Input: part model. Units: mm. Frame: model coordinates. A direction names the side the tool comes from. Coordinates: 2 decimals unless noted, no trailing zeros. Write each loop counter-clockwise with the first axis right and the second up, starting at its lowest first coordinate (ties: lowest second). Pieces come first, ordered by that corner, then holes. Notation, with made-up numbers: (75.25, -18) - (85.25, -18) arc R20 cw to (85.25, 1) - close; hole circle Ø8 at (-32.75, -38). An arc over 180 degrees is marked (long way). Put each result on its own line as item: value. Start each with the question number.
1. Cut plane A-A, the plane x = -21.25. Return loops of the section in (y, z).
2. Access query for faces 5 (the flat face through (-45, 40.364, 1)), 6 (the flat face through (-26.813, 36.211, 0.986)), 7 (the flat face through (-30.617, 37.276, 0.986)). Directions: +Z, -Z, +X, -X, +Y, -Y. A direction counts if a zero-diameter tool reaches every point of the face in a straight line with its end or side. Return the directions, or none.
3. Cut plane B-B, the plane z = 0.7. Count the separate pieces of the cut face and the enclosed holes in it, and give its area (3 significant figures).
4. Pull-direction query (Y, two-part tool) for faces 1 (the flat face through (-30, 34, 0)), 2 (the flat face through (-31, 32.172, 1)), 3 (the flat face through (-23.75, 34.6, 0.99)), 4 (the flat face through (-37.9, 36.33, 0.99)); classes: released by +Y, released by -Y, zero draft, split by the parting line, or undercut.
5. Pin query (flat end, axial travel): pin 1 (1 mm diameter, centred on y = 36, z = 1.5, fed in from +X); pin 2 (1 mm diameter, centred on x = -42.5, y = 37.5, fed in from -Z). Return the tip coordinate at first contact, or that it passes through.
6. Cut plane D-D, the plane x = -30.5. Return loops of the section in (y, z).
7. Line query: line 1 (X direction, y = 39.25, z = 0.6); line 2 (Y direction, x = -43, z = 0.4); line 3 (X direction, y = 31.5, z = 0.9). Output: solid intervals per line, ascending.
from build123d import *

# Parameters (mm, degrees)
BOSS_EXTRUDE1_DEPTH = 2


with BuildPart() as part:
    # Sketch1 → Boss-Extrude1 (new body)
    with BuildSketch(Plane.XY):
        with BuildLine():
            Line((-18.745582546, 31.006914048), (-21.79105099, 40.364252392))
            Line((-21.79105099, 40.364252392), (-23.123022137, 40.364252392))
            Line((-23.123022137, 40.364252392), (-25.740106044, 32.171592169))
            Line((-25.740106044, 32.171592169), (-28.102880037, 32.171592169))
            Line((-28.102880037, 32.171592169), (-25.485755278, 40.364252392))
            Line((-25.485755278, 40.364252392), (-26.78426782, 40.364252392))
            Line((-26.78426782, 40.364252392), (-28.598181785, 34.273274652))
            add(Edge.make_bspline(
                [(-28.598181785, 34.273274652), (-28.792274379, 33.597239241), (-28.906090832, 33.19565427), (-29.126942139, 32.251909163)],
                knots=[6, 6, 6, 6, 7, 7, 7, 7], degree=3))
            add(Edge.make_bspline(
                [(-29.126942139, 32.251909163), (-29.414792363, 33.316129761), (-29.448250968, 33.490163533), (-29.695901842, 34.273274652)],
                knots=[7, 7, 7, 7, 8, 8, 8, 8], degree=3))
            Line((-29.695901842, 34.273274652), (-31.563333235, 40.364252392))
            Line((-31.563333235, 40.364252392), (-32.861845777, 40.364252392))
            Line((-32.861845777, 40.364252392), (-30.197903482, 32.171592169))
            Line((-30.197903482, 32.171592169), (-32.614194903, 32.171592169))
            Line((-32.614194903, 32.171592169), (-35.278137198, 40.364252392))
            Line((-35.278137198, 40.364252392), (-36.610149199, 40.364252392))
            Line((-36.610149199, 40.364252392), (-39.227233105, 32.171592169))
            Line((-39.227233105, 32.171592169), (-40.519045756, 32.171592169))
            add(Edge.make_bspline(
                [(-40.519045756, 32.171592169), (-40.257995098, 32.593235961), (-40.110760894, 33.122037168), (-40.110760894, 33.69765591)],
                knots=[16, 16, 16, 16, 17, 17, 17, 17], degree=3))
            add(Edge.make_bspline(
                [(-40.110760894, 33.69765591), (-40.110760894, 34.82213468), (-40.572604036, 35.511569875), (-41.583307207, 35.913154846)],
                knots=[17, 17, 17, 17, 18, 18, 18, 18], degree=3))
            add(Edge.make_bspline(
                [(-41.583307207, 35.913154846), (-40.739937916, 36.374997988), (-40.365111659, 37.010874903), (-40.365111659, 37.947920118)],
                knots=[18, 18, 18, 18, 19, 19, 19, 19], degree=3))
            add(Edge.make_bspline(
                [(-40.365111659, 37.947920118), (-40.365111659, 38.764530696), (-40.679679744, 39.433866215), (-41.261998378, 39.842151078)],
                knots=[19, 19, 19, 19, 20, 20, 20, 20], degree=3))
            add(Edge.make_bspline(
                [(-41.261998378, 39.842151078), (-41.790799584, 40.23707701), (-42.353018543, 40.364252392), (-43.477497314, 40.364252392)],
                knots=[20, 20, 20, 20, 21, 21, 21, 21], degree=3))
            Line((-43.477497314, 40.364252392), (-46.817515873, 40.364252392))
            Line((-46.817515873, 40.364252392), (-46.817515873, 31.006914048))
            Line((-46.817515873, 31.006914048), (-18.745582546, 31.006914048))
        make_face()
        with BuildLine():
            Line((-43.142829554, 32.171592169), (-45.652837753, 32.171592169))
            Line((-45.652837753, 32.171592169), (-45.652837753, 35.257219109))
            Line((-45.652837753, 35.257219109), (-43.008995132, 35.257219109))
            add(Edge.make_bspline(
                [(-43.008995132, 35.257219109), (-41.958133464, 35.257219109), (-41.362415047, 34.708359081), (-41.362415047, 34.051267898), (-41.362415047, 33.725531232), (-41.362415054, 33.724414624)],
                knots=[0, 0, 0, 0, 1, 2, 2.003439864, 2.003439864, 2.003439864, 2.003439864], degree=3))
            add(Edge.make_bspline(
                [(-41.362415054, 33.724414624), (-41.362417047, 33.400922858), (-41.363577782, 32.75955684), (-42.038450458, 32.171592169), (-43.142829554, 32.171592169)],
                knots=[2.003439864, 2.003439864, 2.003439864, 2.003439864, 3, 4, 4, 4, 4], degree=3))
        make_face(mode=Mode.SUBTRACT)
        with BuildLine():
            Line((-33.87924884, 32.171592169), (-37.955479277, 32.171592169))
            Line((-37.955479277, 32.171592169), (-36.489632855, 37.091191897))
            add(Edge.make_bspline(
                [(-36.489632855, 37.091191897), (-36.295540261, 37.767227308), (-36.181764662, 38.17551217), (-35.960872501, 39.112598239)],
                knots=[1, 1, 1, 1, 2, 2, 2, 2], degree=3))
            add(Edge.make_bspline(
                [(-35.960872501, 39.112598239), (-35.679763022, 38.048336787), (-35.639604525, 37.881002907), (-35.391953651, 37.091191897)],
                knots=[2, 2, 2, 2, 3, 3, 3, 3], degree=3))
            Line((-35.391953651, 37.091191897), (-33.87924884, 32.171592169))
        make_face(mode=Mode.SUBTRACT)
        with BuildLine():
            add(Edge.make_bspline(
                [(-22.47374544, 39.112598239), (-22.19263596, 38.048336787), (-22.152477463, 37.881002907), (-21.904826589, 37.091191897)],
                knots=[1, 1, 1, 1, 2, 2, 2, 2], degree=3))
            Line((-21.904826589, 37.091191897), (-20.392121778, 32.171592169))
            Line((-20.392121778, 32.171592169), (-24.47509296, 32.171592169))
            Line((-24.47509296, 32.171592169), (-23.009246538, 37.091191897))
            add(Edge.make_bspline(
                [(-23.009246538, 37.091191897), (-22.808413199, 37.767227308), (-22.6946376, 38.17551217), (-22.47374544, 39.112598239)],
                knots=[0, 0, 0, 0, 1, 1, 1, 1], degree=3))
        make_face(mode=Mode.SUBTRACT)
        with BuildLine():
            Line((-45.652837753, 36.348239275), (-45.652837753, 39.199615125))
            Line((-45.652837753, 39.199615125), (-43.336963001, 39.199615125))
            add(Edge.make_bspline(
                [(-43.336963001, 39.199615125), (-42.7278448, 39.199615125), (-42.37024646, 39.09102995), (-42.179170008, 38.931701151), (-42.093373815, 38.855654373)],
                knots=[0, 0, 0, 0, 1, 1.908075185, 1.908075185, 1.908075185, 1.908075185], degree=3))
            add(Edge.make_bspline(
                [(-42.093373815, 38.855654373), (-42.083891518, 38.847731554), (-42.074504957, 38.839663032), (-42.065209172, 38.831447907)],
                knots=[1.967701589, 1.967701589, 1.967701589, 1.967701589, 2, 2, 2, 2], degree=3))
            add(Edge.make_bspline(
                [(-42.065209172, 38.831447907), (-42.05671789, 38.823784642), (-42.048329136, 38.815980397), (-42.040044694, 38.808039137)],
                knots=[2, 2, 2, 2, 2.030943823, 2.030943823, 2.030943823, 2.030943823], degree=3))
            add(Edge.make_bspline(
                [(-42.040044694, 38.808039137), (-41.956028804, 38.732525824), (-41.785347703, 38.570931339), (-41.623764076, 38.189616071), (-41.623466502, 37.918150912), (-41.623465709, 37.780586238)],
                knots=[2.097742568, 2.097742568, 2.097742568, 2.097742568, 3, 4, 4.994650719, 4.994650719, 4.994650719, 4.994650719], degree=3))
            add(Edge.make_bspline(
                [(-41.623465709, 37.780586238), (-41.623465704, 37.779846409), (-41.623465704, 37.640790138), (-41.623465704, 37.358942446), (-41.777399801, 36.970716406), (-41.969272715, 36.801149228), (-42.065209172, 36.71636564)],
                knots=[4.994650719, 4.994650719, 4.994650719, 4.994650719, 5, 6, 7, 8, 8, 8, 8], degree=3))
            add(Edge.make_bspline(
                [(-42.065209172, 36.71636564), (-42.161145629, 36.631582051), (-42.353018543, 36.462014874), (-42.7278448, 36.348239275), (-43.336963001, 36.348239275)],
                knots=[8, 8, 8, 8, 9, 10, 10, 10, 10], degree=3))
            Line((-43.336963001, 36.348239275), (-45.652837753, 36.348239275))
        make_face(mode=Mode.SUBTRACT)
    extrude(amount=BOSS_EXTRUDE1_DEPTH)


solid = part.part
Report:
1. outline: (31.01, 0) - (32.17, 0) - (32.17, 2) - (31.01, 2) - close; (34.96, 0) - (38.7, 0) - (38.7, 2) - (34.96, 2) - close
2. face 5: +Z, -Z, +X, -X, +Y
2. face 6: +Z, -Z
2. face 7: +Z, -Z, +Y
3. separate pieces: 1
3. enclosed holes: 4
3. area: 117 mm^2
4. face 1: zero draft
4. face 2: undercut
4. face 3: undercut
4. face 4: released by +Y
5. pin 1: stops at x = -20.21
5. pin 2: passes through
6. outline: (31.01, 0) - (32.17, 0) - (32.17, 2) - (31.01, 2) - close; (33.1, 0) - (36.9, 0) - (36.9, 2) - (33.1, 2) - close
7. line 1: x = -46.82 to -40.7, -36.97 to -34.92, -32.5 to -31.22, -27.12 to -25.84, -23.48 to -21.43
7. line 2: y = 31.01 to 32.17, 35.26 to 36.36, 39.19 to 40.35
7. line 3: x = -46.82 to -18.91
